```python
from build123d import *

# Parameters (mm, degrees)
F0_W           = 50.8
F0_H           = 101.6
F1_DEPTH       = 3.175
F2_W           = 3.175
F2_H           = 12.7
F2_H_2         = 19.05
F3_DEPTH       = 6.35
F5_DEPTH       = 101.601
F6_R           = 1.5875
F7_DEPTH       = 101.601
F9_D           = 3.175
F9_CSINK_D     = 6.35
F9_CSINK_ANGLE = 90


with BuildPart() as f1:
    # F0 (on Front) → F1 (new body)
    with BuildSketch(Plane.XZ):
        Rectangle(F0_W, F0_H)
    extrude(amount=F1_DEPTH)

    # F2 (on face) → F3 (join)
    with BuildSketch(Plane(origin=(-25.4, 0, 0), x_dir=(0, -1, 0), z_dir=(-1, 0, 0))):
        with Locations((-1.5875, 0)):
            Rectangle(F2_W, F2_H)
        with Locations((-1.5875, -41.275)):
            Rectangle(F2_W, F2_H_2)
        with Locations((1.5875, 41.275)):
            Rectangle(F2_W, F2_H_2)
        with Locations((1.5875, -41.275)):
            Rectangle(F2_W, F2_H_2)
        with Locations((1.5875, 0)):
            Rectangle(F2_W, F2_H)
        with Locations((-1.5875, 41.275)):
            Rectangle(F2_W, F2_H_2)
    extrude(amount=F3_DEPTH)

    # F4 (on face) → F5 (cut, through all)
    with BuildSketch(Plane.XY.offset(50.8)):
        with BuildLine():
            ThreePointArc((-31.75, -3.5e-09), (-30.8200640315, 2.245064029), (-28.575, 3.175))
            Line((-28.575, 3.175), (-31.75, 3.175))
            Line((-31.75, 3.175), (-31.75, -3.5e-09))
        make_face()
        with BuildLine():
            ThreePointArc((-28.575, 3.175), (-26.3299359697, 2.2450640303), (-25.4, 0))
            Line((-25.4, 0), (-25.4, 3.175))
            Line((-25.4, 3.175), (-28.575, 3.175))
        make_face()
        with BuildLine():
            Line((-31.75, -3.175), (-28.575, -3.175))
            ThreePointArc((-28.575, -3.175), (-30.820064029, -2.2450640315), (-31.75, -3.5e-09))
            Line((-31.75, -3.5e-09), (-31.75, -3.175))
        make_face()
    extrude(amount=-F5_DEPTH, mode=Mode.SUBTRACT)

    # F6 (on face) → F7 (cut, through all)
    with BuildSketch(Plane.XY.offset(50.8)):
        with Locations((-28.575, 0)):
            Circle(F6_R)
    extrude(amount=-F7_DEPTH, mode=Mode.SUBTRACT)

    # F9 (through all)
    with Locations(Plane(origin=(0, 0, 0), x_dir=(-1, 0, 0), z_dir=(0, 1, 0))):
        with Locations((-19.05, 38.1), (-19.05, 0), (-19.05, -38.1)):
            CounterSinkHole(F9_D / 2, F9_CSINK_D / 2, counter_sink_angle=F9_CSINK_ANGLE)


solid = f1.part
```
Check sheet for the modelled part. Datum: model origin and axes. Units: mm. A direction names the side the tool comes from. Coordinates: 2 decimals unless noted, no trailing zeros. Write each loop counter-clockwise with the first axis right and the second up, starting at its lowest first coordinate (ties: lowest second). Pieces come first, ordered by that corner, then holes. Notation, with made-up numbers: M -16.75,-32.75 L 24.25,-32.75 A22 cw 24.25,-12.75 Z; hole C 9.25,-9 d8. An arc over 180 degrees is marked long. Write item = value, one per line. Start each with the question number.
1. Tool access check on faces 1 (the flat face through (-27, -1, 6.35)), 2 (the cylindrical face through (-27.06, 0.48, 41.41)), 3 (the flat face through (0, 0, 1)). Record the directions out of +Z, -Z, +X, -X, +Y, -Y that give a thin tool (end or side, any length) a straight path to the whole face; none if there is none.
2. Mould release check, pull along Z, two halves, no side actions. Record for faces 4 (the flat face through (-27, -1, -31.75)), 5 (the flat face through (-4, -1, 50.8)), 6 (the flat face through (-1, -3.175, -1)), 7 (the flat face through (-25.4, -2, -19)): pulls with the +Z half, pulls with the -Z half, needs draft (parallel to the pull), parting line crosses it, or undercut.
3. Sectioned sample at D-D (z = -26). Record the cut outline in (x, y) (3 decimals).
4. Go/stop test with flat-tipped pins: pin 1 (3.5 mm diameter, centred on x = 19.05, z = 38.1, fed in from +Y) (3 decimals); pin 2 (2 mm diameter, centred on x = -6, z = 26, fed in from +Y); pin 3 (2.5 mm diameter, centred on y = -2, z = 19, fed in from -X). Record where each tip stops, or that it passes through.
5. Sectioned sample at B-B (x = 19.05). Record the cut outline in (y, z) (1 decimal), then the cut area to 3 significant figures.
6. Sectioned sample at C-C (x = -2.5). Record the cut outline in (y, z) (3 decimals), then the cut area to 3 significant figures.
7. Sectioned sample at A-A (z = 38.1). State how many separate pieces and enclosed holes the cut face has, then the cut area to 3 significant figures.
8. Thickness scan on probe 1 along Z at (x, y) = (-27.5, -1.75); probe 2 along Z at (x, y) = (19.05, -1.95); probe 3 along X at (y, z) = (-0.25, 10). Record the ranges inside material, lowest first.
The answers:
q1.face_1 = -X, +Y, -Y
q1.face_2 = +Z, -Z
q1.face_3 = +Z, -Z, +X, +Y
q2.face_4 = undercut
q2.face_5 = pulls with the +Z half
q2.face_6 = needs draft
q2.face_7 = undercut
q3.outline = M -25.4,-3.175 L 25.4,-3.175 L 25.4,0 L -25.4,0 Z
q4.pin_1 = -1.425
q4.pin_2 = 0
q4.pin_3 = -25.4
q5.outline = M -3.2,-50.8 L 0,-50.8 L 0,-41.3 L -1.6,-39.7 L -3.2,-39.7 Z; M -3.2,-36.5 L -1.6,-36.5 L 0,-34.9 L 0,-3.2 L -1.6,-1.6 L -3.2,-1.6 Z; M -3.2,1.6 L -1.6,1.6 L 0,3.2 L 0,34.9 L -1.6,36.5 L -3.2,36.5 Z; M -3.2,39.7 L -1.6,39.7 L 0,41.3 L 0,50.8 L -3.2,50.8 Z
q5.area = 285 mm²
q6.outline = M -3.175,-50.8 L 0,-50.8 L 0,50.8 L -3.175,50.8 Z
q6.area = 323 mm²
q7.separate_pieces = 2
q7.enclosed_holes = 1
q7.area = 175 mm²
q8.probe_1 = -50.8 to -31.75, -6.35 to 6.35, 31.75 to 50.8
q8.probe_2 = -50.8 to -39.69, -36.51 to -1.59, 1.59 to 36.51, 39.69 to 50.8
q8.probe_3 = -25.4 to 25.4
